Autodesk Inventor part; units mm, degrees
ref_plane "YZ Plane" through (0, 0, 0) normal (1, 0, 0) x (0, 1, 0)
ref_plane "XZ Plane" through (0, 0, 0) normal (0, 1, 0) x (-1, 0, 0)
ref_plane "XY Plane" through (0, 0, 0) normal (0, 0, 1) x (1, 0, 0)
sketch "Sketch1" plane through (0, 0, 0) normal (0, 0, 1) x (1, 0, 0)
  line L0 (-3.5818, 0) -> (-9.2068, 0)
  line L1 (-9.2068, 0) -> (-6.3943, 4.8714)
  line L2 (-6.3943, 4.8714) -> (-0.7693, 4.8714)
  line L3 (-0.7693, 4.8714) -> (2.0432, 0)
  line L4 (2.0432, 0) -> (-0.7693, -4.8714)
  line L5 (-0.7693, -4.8714) -> (-6.3943, -4.8714)
  line L6 (-6.3943, -4.8714) -> (-9.2068, 0)
  point P0 (-0.7818, 0)
  dimension "d0" = 5.625
extrude "Extrusion1" add sketch "Sketch1" along normal blind 6.3
sketch "Sketch2" plane through (0, 0, 6.3) normal (0, 0, 1) x (1, 0, 0)
  circle A0 centre (-2.8, 0) radius 2.5
  circle A1 centre (-2.8, 0) radius 3.5
  point P0 (0, 0)
  dimension "d3" = 7
extrude "Extrusion2" add sketch "Sketch2" along normal blind 2.7
sketch "Sketch3" plane through (-2.8, 0, 6.3) normal (0, 0, 1) x (1, 0, 0)
  circle A0 centre (0, 0) radius 2.5
  point P0 (2.8, 0)
extrude "Extrusion3" cut sketch "Sketch3" against normal through all
properties part number "Eccentric Spacer"
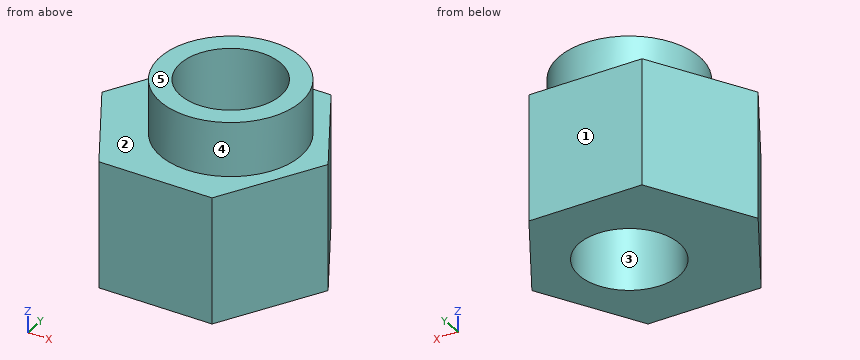
Build history of the part. All positions in model axes, mm. Face numbers are marked on the shaded views. A direction names the side the tool comes from. Give positions to 0.01 mm unless a question says otherwise; leave off trailing zeros. Order: outer loops, then holes, each group sorted by start corner. A loop starts at its lowest first (then second) coordinate and runs counter-clockwise, first axis right, second up. Notation, with made-up numbers: M 81.5,-7 L 115.5,-7 A32 cw 115.5,28 Z; hole C 31.25,-33.5 d7. An arc over 180 degrees is marked long. Put each result on its own line as item: value.
Item 1: Slice it at D-D, the plane z = 7.75. Write the cut outline in (x, y).
From the geometry:
outline: C -2.8,0 d7; hole C -2.8,0 d5
Item 2: Probe line 1 (Z direction, x = -1.25, y = 4.25); line 2 (Y direction, x = -2.8, z = 4.75); line 3 (X direction, y = -0.75, z = 8). List the from-to ranges inside material, lowest first. Write a range as [from, to].
From the geometry:
line 1: z = [0, 6.3]
line 2: y = [-4.87, -2.5], [2.5, 4.87]
line 3: x = [-6.22, -5.18], [-0.42, 0.62]
Item 3: Flat gauge pins, fed straight in: pin 1 Ø1 at (y, z) = (1, 4) entering from +X; pin 2 Ø4 at (x, y) = (-2.8, 0) entering from +Z; pin 3 Ø4 at (x, y) = (-7.5, 3) entering from +Z; pin 4 Ø3 at (x, z) = (-0.5, 2) entering from -Y. Where does each tip first touch, or does it go through?
From the geometry:
pin 1: stops at x = 1.75
pin 2: passes through
pin 3: stops at z = 6.3
pin 4: stops at y = -4.87
Item 4: Slice it at B-B, the plane y = -1.25. Write the cut outline in (x, z).
From the geometry:
outline: M -8.49,0 L -4.97,0 L -4.97,9 L -6.07,9 L -6.07,6.3 L -8.49,6.3 Z; M -0.63,0 L 1.32,0 L 1.32,6.3 L 0.47,6.3 L 0.47,9 L -0.63,9 Z
Item 5: Two-plate mould, pull along Y, no slides. Class the marked faces 1, 2 and 3: +Y half, -Y half, draft (parallel to the pull), parting line (faces both ways), or undercut.
From the geometry:
face 1: +Y half
face 2: draft
face 3: undercut
Item 6: 3-axis set-ups, long thin cutter, end or side, ignore diameter. For the marked faces 4 and 5: which of +Z, -Z, +X, -X, +Y, -Y reach the whole face in a straight line?
From the geometry:
face 4: +Z
face 5: +Z, +X, -X, +Y, -Y
Item 7: Slice it at A-A, the plane x = -2.8. Write the cut outline in (y, z), plus the area to 3 significant figures.
From the geometry:
outline: M -4.87,0 L -2.5,0 L -2.5,9 L -3.5,9 L -3.5,6.3 L -4.87,6.3 Z; M 2.5,0 L 4.87,0 L 4.87,6.3 L 3.5,6.3 L 3.5,9 L 2.5,9 Z
area: 35.3 mm2
Item 8: Slice it at C-C, the plane z = 3. Write the cut outline in (x, y), plus the area to 3 significant figures.
From the geometry:
outline: M -9.21,0 L -6.39,-4.87 L -0.77,-4.87 L 2.04,0 L -0.77,4.87 L -6.39,4.87 Z; hole C -2.8,0 d5
area: 62.6 mm2
